Input: part model. Units: mm. Frame: model coordinates. Face numbers are marked on the shaded views. A direction names the side the tool comes from. Give positions to 0.01 mm unless a question says otherwise; leave off trailing zeros. Loops run counter-clockwise (first coordinate to the right, second up) from the corner with the lowest first, then second, coordinate; pieces in that order, holes last. Notation, with made-up numbers: (89, 83.25) - (96, 83.25) arc R30 ccw to (96, 115.25) - close; hole circle Ø8 at (-9, 38). An arc over 180 degrees is marked (long way). Answer as a JSON object with one key per item and string values. Group by question number.
(1) Section query A-A (y = 0). Return loops of the section in (x, z), plus the area to 3 significant figures.
(2) Access query for the marked faces 5, 6 and 7. Directions: +Z, -Z, +X, -X, +Y, -Y. A direction counts if a zero-diameter tool reaches every point of the face in a straight line with its end or side. Return the directions, or none.
(3) Section query C-C (z = 0.3). Return loops of the section in (x, y), plus the area to 3 significant figures.
(4) Material intervals for L1, parallel to X at y = 0, z = 0.8; L2, parallel to X at y = 9.25, z = 0.8; L3, parallel to X at y = -8.5, z = -1.95, sorted ascending.
(5) Pin query (flat end, axial travel): P1, Ø1.5, axis at y = 8, z = 1, coming from the +X side; P2, Ø1, axis at x = -9, z = 1, coming from the +Y side. Return the tip coordinate at first contact, or that it passes through.
(6) Mould query, pull axis X, two halves, no side actions, for the marked faces 1, 2, 3 and 4. Classes: +X half, -X half, draft (parallel to the pull), parting line (faces both ways), or undercut.
(7) Section query B-B (y = 9.5). Return loops of the section in (x, z).
(8) Section query D-D (y = -7). Return loops of the section in (x, z), plus the area to 3 significant figures.
```python
from build123d import *

# Parameters (mm, degrees)
PAD_DEPTH    = 2.5
SKETCH003_R  = 10.5
POCKET_DEPTH = 5


with BuildPart() as part:
    # Sketch → Pad (new body, symmetric)
    with BuildSketch(Plane.XY):
        with BuildLine():
            ThreePointArc((8.786596, -8.172865), (11.99665, -0.28352), (9.162874, 7.74866))
            Line((11.290112, 9.875898), (9.162874, 7.74866))
            Line((9.875898, 11.290112), (11.290112, 9.875898))
            Line((7.74866, 9.162874), (9.875898, 11.290112))
            ThreePointArc((7.74866, 9.162874), (0, 12), (-7.74866, 9.162874))
            Line((-7.74866, 9.162874), (-9.875898, 11.290112))
            Line((-9.875898, 11.290112), (-11.290112, 9.875898))
            Line((-11.290112, 9.875898), (-9.162874, 7.74866))
            ThreePointArc((-9.162874, 7.74866), (-11.99665, -0.28352), (-8.786596, -8.172865))
            Line((-8.786596, -8.172865), (-10.63343, -10.579705))
            Line((-10.63343, -10.579705), (-9.131421, -11.9003))
            Line((0, 0), (-9.131421, -11.9003))
            Line((0, 0), (9.131421, -11.9003))
            Line((9.131421, -11.9003), (10.63343, -10.579705))
            Line((10.63343, -10.579705), (8.786596, -8.172865))
        make_face()
    extrude(amount=PAD_DEPTH, both=True)

    # Sketch003 → Pocket (cut)
    with BuildSketch(Plane.XY.offset(2.5)):
        Circle(SKETCH003_R)
    extrude(amount=-POCKET_DEPTH, mode=Mode.SUBTRACT)


solid = part.part
```
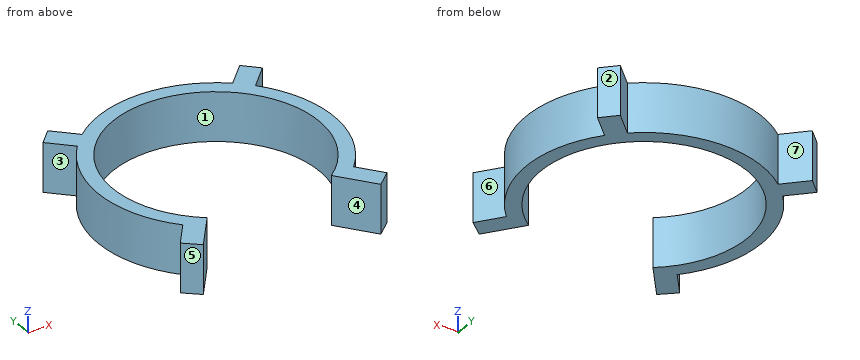
Recorded:
{
 "1": {"outline": "(-12, -2.5) - (-10.5, -2.5) - (-10.5, 2.5) - (-12, 2.5) - close; (10.5, -2.5) - (12, -2.5) - (12, 2.5) - (10.5, 2.5) - close", "area": "15.0 mm^2"},
 "2": {"face 5": "+Z, -Z, -X, -Y", "face 6": "+Z, -Z, +X", "face 7": "+Z, -Z, +Y"},
 "3": {"outline": "(-11.29, 9.88) - (-9.16, 7.75) arc R12 ccw to (-8.79, -8.17) - (-10.63, -10.58) - (-9.13, -11.9) - (-6.39, -8.33) arc R10.5 cw (long way) to (6.39, -8.33) - (9.13, -11.9) - (10.63, -10.58) - (8.79, -8.17) arc R12 ccw to (9.16, 7.75) - (11.29, 9.88) - (9.88, 11.29) - (7.75, 9.16) arc R12 ccw to (-7.75, 9.16) - (-9.88, 11.29) - close", "area": "108 mm^2"},
 "4": {"L1": "x = -12 to -10.5, 10.5 to 12", "L2": "x = -10.66 to -7.84, -7.64 to -4.97, 4.97 to 7.64, 7.84 to 10.66", "L3": "x = -9.04 to -6.52, 6.52 to 9.04"},
 "5": {"P1": "stops at x = 10.16", "P2": "stops at y = 10.91"},
 "6": {"face 1": "undercut", "face 2": "+X half", "face 3": "-X half", "face 4": "undercut"},
 "7": {"outline": "(-10.91, -2.5) - (-8.09, -2.5) - (-8.09, 2.5) - (-10.91, 2.5) - close; (-7.33, -2.5) - (-4.47, -2.5) - (-4.47, 2.5) - (-7.33, 2.5) - close; (4.47, -2.5) - (7.33, -2.5) - (7.33, 2.5) - (4.47, 2.5) - close; (8.09, -2.5) - (10.91, -2.5) - (10.91, 2.5) - (8.09, 2.5) - close"},
 "8": {"outline": "(-9.75, -2.5) - (-7.83, -2.5) - (-7.83, 2.5) - (-9.75, 2.5) - close; (7.83, -2.5) - (9.75, -2.5) - (9.75, 2.5) - (7.83, 2.5) - close", "area": "19.2 mm^2"}
}
